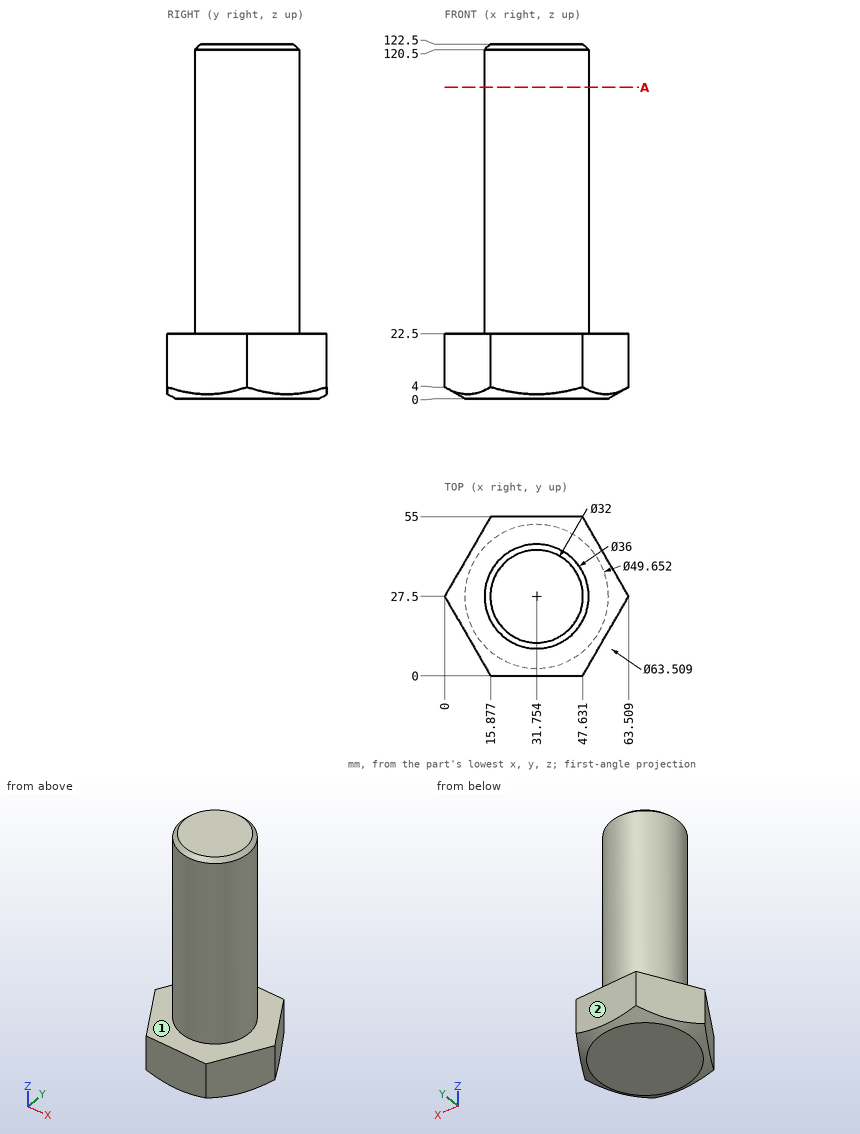
Study the drawing (mm; zero at the part's minimum x, y, z) and answer. A direction names the side the tool comes from. Give positions to 0.01 mm unless a question says otherwise; leave off trailing zeros. Write each loop counter-clockwise with the first axis right and the second up, starting at its lowest first coordinate (ties: lowest second). Pieces come first, ordered by that corner, then holes. Notation, with made-up numbers: (21.5, 19.5) -> (55.5, 19.5) arc R22 ccw to (55.5, 42.5) -> close; hole circle Ø9 at (89.25, 47). An arc over 180 degrees is marked (long way). Answer as a JSON object with one key per item and string values. Group by question number.
1) Consider L1, parallel to Z at x = 46.5, y = 43; L2, parallel to Y at x = 40, z = 109; L3, parallel to Z at x = 47, y = 48.5. Determine where each line is inside the solid, lowest interval first. Write a range as from..to.
2) Each of these flat-tipped pins is pushed along its axis until it touches: P1, Ø2, axis at x = 30, z = 89.5, coming from the +Y side; P2, Ø1, axis at x = 43, z = 35.5, coming from the -Y side; P3, Ø2, axis at y = 13.5, z = 29.5, coming from the -X side (1 decimal). Where does it stop, or does it pass through?
3) Find section A-A (z = 107.5). Write down the section's boundary in (x, y) (1 decimal).
4) A tool of negligible diameter and unlimited length cuts with its end or side. For the marked faces 1 and 2, from which of +Z, -Z, +X, -X, +Y, -Y can it reach the whole face along a straight path? Write none if from no direction.
Values follow:
{
 "1": {"L1": "z = 0..22.5", "L2": "y = 11.5..43.5", "L3": "z = 0.65..22.5"},
 "2": {"P1": "stops at y = 45.48", "P2": "stops at y = 13.06", "P3": "stops at x = 19.3"},
 "3": {"outline": "circle Ø36 at (31.8, 27.5)"},
 "4": {"face 1": "+Z", "face 2": "+Z, -Z, +X, -X, +Y"}
}
